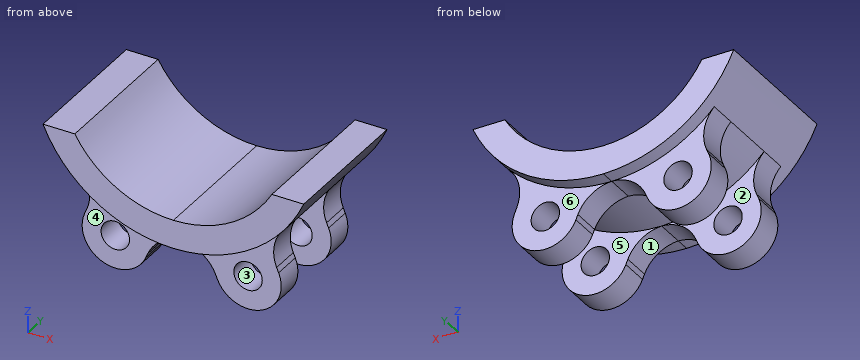
from build123d import *

# Parameters (mm, degrees)
BOSS_EXTRU_1_DEPTH           = 7.5
ESQUISSE2_R                  = 1.5
BOSS_EXTRU_2_DEPTH           = 6
CONG_2_R                     = 4
CONG_2_OF_SYM_TRIE1_R        = 4
ENL_V_MAT_EXTRU_1_DEPTH      = 3
ENL_V_MAT_EXTRU_1_DEPTH_BACK = 3
ESQUISSE3_R                  = 23.003278447
ESQUISSE3_R_2                = 15


with BuildPart() as part:
    # Esquisse1 → Boss.-Extru.1 (new, symmetric)
    with BuildSketch(Plane(origin=(0, 0, 0), x_dir=(1, 0, 0), z_dir=(0, 1, 0))):
        with BuildLine():
            Line((0, 15), (0, 12))
            ThreePointArc((0, 12), (-6, 10.392304845), (-10.392304845, 6))
            Line((-10.392304845, 6), (-13.747727085, 6))
            ThreePointArc((-13.747727085, 6), (-8.215838363, 12.549900398), (0, 15))
        make_face()
    boss_extru_1 = extrude(amount=BOSS_EXTRU_1_DEPTH, both=True)

    # Esquisse2 → Boss.-Extru.2 (add, symmetric)
    with BuildSketch(Plane(origin=(0, 0, 0), x_dir=(1, 0, 0), z_dir=(0, 1, 0))):
        with BuildLine():
            Line((-10.224496324, 15.222012841), (-8.896811047, 12.07670291))
            ThreePointArc((-8.896811047, 12.07670291), (-5.833333333, 13.81926996), (-2.447818399, 14.798925133))
            Line((-2.447818399, 14.798925133), (-3.775503676, 17.944235063))
            ThreePointArc((-3.775503676, 17.944235063), (-8.361111111, 19.807620276), (-10.224496324, 15.222012841))
        make_face()
        with Locations(Location((-7, 16.583123952, 0), (0, 0, 270))):
            Circle(ESQUISSE2_R, mode=Mode.SUBTRACT)
    boss_extru_2 = extrude(amount=BOSS_EXTRU_2_DEPTH, both=True)

    # Congé2
    # the kernel refuses this fillet: 4 mm, written as the material it adds along each edge
    with BuildSketch(Plane(origin=(-2.447818399, -6, -14.798925133), x_dir=(0.9966431178830178, 0, -0.0818687704586858), z_dir=(0, 1, 0))) as cong_2_piece_1:
        with BuildLine():
            CenterArc((2.904362046, 3.974799123), CONG_2_R, 198.189389649, 65.375681648)
            Line((-0.895757454, 2.726163155), (-0.971759844, 2.701190435))
            Line((-0.971759844, 2.701190435), (-0.07600239, -0.024972719))
            Line((-0.07600239, -0.024972719), (0.006549502, -0.079731449))
            ThreePointArc((0.006549502, -0.079731449), (1.228031557, -0.029646768), (2.447097135, -0.079495982))
            Line((2.447097135, -0.079495982), (2.456063114, 0))
        make_face()
    extrude(amount=12)
    with BuildSketch(Plane(origin=(-8.896811047, -6, -12.07670291), x_dir=(-0.7517608452817168, 0, 0.6594358433549989), z_dir=(0, 1, 0))) as cong_2_piece_2:
        with BuildLine():
            CenterArc((2.891216238, -3.985511596), CONG_2_R, 94.878081885, 66.750437409)
            Line((-0.904915803, -2.724804838), (-0.980838444, -2.699590703))
            Line((-0.980838444, -2.699590703), (-0.075922641, 0.025214135))
            Line((-0.075922641, 0.025214135), (0.006802862, 0.079710232))
            ThreePointArc((0.006802862, 0.079710232), (1.275536575, 0.025668484), (2.544270289, 0.079710232))
            Line((2.544270289, 0.079710232), (2.551073151, 0))
        make_face()
    extrude(amount=12)

    # Symétrie1: Boss.-Extru.1, Boss.-Extru.2 across plane
    add(boss_extru_1.mirror(Plane(origin=(0, -7.5, -15), x_dir=(0, 0, 1), z_dir=(1, 0, 0))))
    add(boss_extru_2.mirror(Plane(origin=(0, -7.5, -15), x_dir=(0, 0, 1), z_dir=(1, 0, 0))))

    # Congé2 of Symétrie1
    # the kernel refuses this fillet: 4 mm, written as the material it adds along each edge
    with BuildSketch(Plane(origin=(2.447818399, -6, -14.798925133), x_dir=(-0.9966431178830035, 0, -0.08186877045886062), z_dir=(0, 1, 0))) as cong_2_of_sym_trie1_piece_1:
        with BuildLine():
            CenterArc((2.904362046, -3.974799123), CONG_2_OF_SYM_TRIE1_R, 96.434928703, 65.375681648)
            Line((-0.895757454, -2.726163155), (-0.971759844, -2.701190435))
            Line((-0.971759844, -2.701190435), (-0.07600239, 0.024972719))
            Line((-0.07600239, 0.024972719), (0.006549502, 0.079731449))
            ThreePointArc((0.006549502, 0.079731449), (1.228031557, 0.029646768), (2.447097135, 0.079495982))
            Line((2.447097135, 0.079495982), (2.456063114, 0))
        make_face()
    extrude(amount=12)
    with BuildSketch(Plane(origin=(8.896811047, -6, -12.07670291), x_dir=(0.7517608452817176, 0, 0.6594358433549979), z_dir=(0, 1, 0))) as cong_2_of_sym_trie1_piece_2:
        with BuildLine():
            CenterArc((2.891216238, 3.985511596), CONG_2_OF_SYM_TRIE1_R, 198.371480706, 66.750437409)
            Line((-0.904915803, 2.724804838), (-0.980838444, 2.699590703))
            Line((-0.980838444, 2.699590703), (-0.075922641, -0.025214135))
            Line((-0.075922641, -0.025214135), (0.006802862, -0.079710232))
            ThreePointArc((0.006802862, -0.079710232), (1.275536575, -0.025668484), (2.544270289, -0.079710232))
            Line((2.544270289, -0.079710232), (2.551073151, 0))
        make_face()
    extrude(amount=12)

    # Esquisse3 → Enlèv. mat.-Extru.1 (cut, two sides: drawn at the far end of the back side and taken through both)
    with BuildSketch(Plane(origin=(0, 0, 0), x_dir=(1, 0, 0), z_dir=(0, 1, 0)).offset(-ENL_V_MAT_EXTRU_1_DEPTH_BACK)):
        Circle(ESQUISSE3_R)
        Circle(ESQUISSE3_R_2, mode=Mode.SUBTRACT)
    extrude(amount=ENL_V_MAT_EXTRU_1_DEPTH + ENL_V_MAT_EXTRU_1_DEPTH_BACK, mode=Mode.SUBTRACT)


solid = part.part
Build history of the part. All positions in model axes, mm. Face numbers are marked on the shaded views. A direction names the side the tool comes from. Round coordinates to 2 decimals unless told otherwise and drop trailing zeros. Write each loop counter-clockwise with the first axis right and the second up, starting at its lowest first coordinate (ties: lowest second). Pieces come first, ordered by that corner, then holes. Notation, with made-up numbers: M -2.5,88.5 L 4.5,88.5 A17 cw 4.5,109.5 Z; hole C 16,3.25 d5. An arc over 180 degrees is marked long. Answer in a Markdown table with one row per item.
1. Flat gauge pins, fed straight in: P1, Ø5, axis at y = -1.5, z = -16, coming from the +X side; P2, Ø4, axis at x = 7, z = -16.58, coming from the +Y side; P3, Ø3, axis at y = -4, z = -12, coming from the +X side. Where does each tip first touch, or does it go through?
Geometry check:
| item | result |
|---|---|
| P1 | x = 10.5 |
| P2 | y = 6 |
| P3 | x = 10.72 |
2. Saw through at D-D (y = 1). List the corners of the cut face in (x, z).
Geometry check:
| item | result |
|---|---|
| outline | M -13.75,-6 A15 ccw 13.75,-6 L 10.39,-6 A12 cw -10.39,-6 Z |
3. Probe L1, parallel to Y at x = 2.5, z = -15.5; L2, parallel to X at y = -5.75, z = -7; L3, parallel to X at y = -4, z = -7.5. List the from-to ranges inside material, lowest first. Write a range as [from, to].
Geometry check:
| item | result |
|---|---|
| L1 | [-6, -3], [3, 6] |
| L2 | [-13.27, -9.75], [9.75, 13.27] |
| L3 | [-12.99, -9.37], [9.37, 12.99] |
4. Which spindle directions (+Z, -Z, +X, -X, +Y, -Y) get a long thin tool onto all of the face, cutting with end or side? Do the marked faces 4, 5 and 6. Say none if no direction does.
Geometry check:
| item | result |
|---|---|
| face 4 | -Z, -X, -Y |
| face 5 | -Z, +X |
| face 6 | -Z, +X, +Y |
5. Mould opens along Z. For the marked faces 1, 2 and 3 say: +Z half, -Z half, draft (parallel to the pull), parting line (faces both ways), or undercut.
Geometry check:
| item | result |
|---|---|
| face 1 | -Z half |
| face 2 | draft |
| face 3 | undercut |
6. Saw through at A-A (z = -16.5). State how many separate pieces and enclosed holes the cut face has, and give its area (3 significant figures).
Geometry check:
| item | result |
|---|---|
| separate pieces | 8 |
| enclosed holes | 0 |
| area | 54.0 mm2 |
7. Saw through at B-B (x = -7). List the corners of the cut face in (y, z).
Geometry check:
| item | result |
|---|---|
| outline | M -7.5,-13.27 L -6,-13.27 L -6,-15.08 L -3,-15.08 L -3,-13.27 L 3,-13.27 L 3,-15.08 L 6,-15.08 L 6,-13.27 L 7.5,-13.27 L 7.5,-9.75 L -7.5,-9.75 Z; M -6,-20.08 L -3,-20.08 L -3,-18.08 L -6,-18.08 Z; M 3,-20.08 L 6,-20.08 L 6,-18.08 L 3,-18.08 Z |
